```python
from build123d import *

# Parameters (mm, degrees)
F0_W     = 1358.9
F0_H     = 635
F0_H_2   = 939.8
F1_DEPTH = 304.8
F2_DEPTH = 76.2
F3_SIZE2 = 76.19999
F3_SIZE  = 634.99999
F4_W     = 1358.9
F4_H     = 800.1
F5_DEPTH = 25.4


# Not quite as in the source:
# - a fillet or chamfer is up to 0.001 mm smaller than in the source, because OpenCascade refuses the exact size


with BuildPart() as f1:
    # F0 (on Top) → F1 (new body)
    with BuildSketch(Plane.XY):
        with Locations((679.45, 1257.3)):
            Rectangle(F0_W, F0_H)
        with Locations((679.45, 469.9)):
            Rectangle(F0_W, F0_H_2)
    extrude(amount=-F1_DEPTH)

    # F0 (on Top) → F2 (join)
    with BuildSketch(Plane.XY):
        with Locations((679.45, 1257.3)):
            Rectangle(F0_W, F0_H)
    extrude(amount=F2_DEPTH)

    # F3 (size 635 and 76.2 in the source; OpenCascade refuses exactly that, so slightly less here)
    f3_edges = [f1.edges().sort_by_distance(p)[0] for p in [
        (679.45, 939.8, 76.2),
    ]]
    f3_side = f1.faces().sort_by_distance((679.45, 1257.3, 76.2))[0]
    chamfer(f3_edges, length=F3_SIZE, length2=F3_SIZE2, reference=f3_side)

    # F4 (on face) → F5 (join)
    with BuildSketch(Plane.XZ):
        with Locations((679.45, 400.05)):
            Rectangle(F4_W, F4_H)
        with BuildLine():
            Line((1116.8070589646, 12.7), (242.0929410354, 12.7))
            ThreePointArc((242.0929410354, 12.7), (211.2114924509, 23.1642077886), (193.0524806695, 50.2458215227))
            Line((193.0524806695, 50.2458215227), (84.9974320158, 450.0495015416))
            ThreePointArc((84.9974320158, 450.0495015416), (82.0087933028, 466.189437514), (81.6581746464, 482.6))
            ThreePointArc((81.6581746464, 482.6), (83.887579714, 498.5521883341), (88.6100008594, 513.9515811185))
            Line((88.6100008594, 513.9515811185), (184.1425076023, 755.2968613112))
            ThreePointArc((184.1425076023, 755.2968613112), (202.8211285229, 778.6145245993), (231.3766835464, 787.4))
            Line((231.3766835464, 787.4), (1127.5233164536, 787.4))
            ThreePointArc((1127.5233164536, 787.4), (1156.0788714771, 778.6145245993), (1174.7574923977, 755.2968613112))
            Line((1174.7574923977, 755.2968613112), (1270.2899991406, 513.9515811185))
            ThreePointArc((1270.2899991406, 513.9515811185), (1275.012420286, 498.5521883341), (1277.2418253536, 482.6))
            ThreePointArc((1277.2418253536, 482.6), (1276.8912066972, 466.189437514), (1273.9025679842, 450.0495015416))
            Line((1273.9025679842, 450.0495015416), (1165.8475193305, 50.2458215227))
            ThreePointArc((1165.8475193305, 50.2458215227), (1147.6885075491, 23.1642077886), (1116.8070589646, 12.7))
        make_face(mode=Mode.SUBTRACT)
    extrude(amount=-F5_DEPTH)


solid = f1.part
```
Here's how the part is built. I have some questions about the finished solid (model axes, mm). A direction names the side the tool comes from. Give positions to 0.01 mm unless a question says otherwise; leave off trailing zeros. Loops run counter-clockwise (first coordinate to the right, second up) from the corner with the lowest first, then second, coordinate; pieces in that order, holes last. Notation, with made-up numbers: M -22,47.5 L 29,47.5 A13 ccw 29,69.5 Z; hole C 7.5,73 d5. An arc over 180 degrees is marked long. Use one line per item in the form item = value. Start each with the question number.
Q1. If we section it at C-C (y = 543.5): Write out the boundary of the cut face in (x, z).
Q2. Which directions (+Z, -Z, +X, -X, +Y, -Y) give clear straight access to the entire face, cutting with the end or side of a thin tool? Please do faces 4 (the flat face through (670, 798, -304.8)), 5 (the cylindrical face through (1148.06, 12.52, 23.45)), 6 (the flat face through (1221.855, 12.522, 636.314)), 7 (the flat face through (670, 489, 0)).
Q3. Will this pin go through, and if not, where does the flat tip stop? pin 1 Ø8 at (x, y) = (352, 214) entering from +Z.
Q4. If we section it at B-B (z = 723): Write out the boundary of the cut face in (x, y).
Q5. Thinking about a two-plate mould opening in X: for faces 1 (the cylindrical face through (211.582, 12.522, 22.883)), 2 (the flat face through (1358.9, 842, -164)), 3 (the flat face through (670, 1574.8, -117)), which applies, +X half, -X half, draft (parallel to the pull), parting line (faces both ways), or undercut?
Q6. If we section it at D-D (z = 173.5): Write out the boundary of the cut face in (x, y), then the cut area to 3 significant figures.
Q7. I need wall thicknesses on line 1 along Z through (x, y) = (636, 639.5); line 2 along Y through (x, z) = (1242, 286.5); line 3 along Z through (x, y) = (652, 1460). Which ranges of each line are inside material? Lowest first, please.
Taken from the geometry:
q1.outline = M 0,-304.8 L 1358.9,-304.8 L 1358.9,0 L 0,0 Z
q2.face_4 = -Z, +X, -X, +Y, -Y
q2.face_5 = -Y
q2.face_6 = +Y, -Y
q2.face_7 = +Z, +X, -X
q3.pin_1 = 0
q4.outline = M 0,0 L 171.36,0 L 171.36,25.4 L 0,25.4 Z; M 1187.54,0 L 1358.9,0 L 1358.9,25.4 L 1187.54,25.4 Z
q5.face_1 = undercut
q5.face_2 = +X half
q5.face_3 = draft
q6.outline = M 0,0 L 159.74,0 L 159.74,25.4 L 0,25.4 Z; M 1199.16,0 L 1358.9,0 L 1358.9,25.4 L 1199.16,25.4 Z
q6.area = 8,110 mm^2
q7.line_1 = -304.8 to 0
q7.line_2 = 0 to 25.4
q7.line_3 = -304.8 to 62.42
